Check sheet for the drawn part. Datum: minimum x, y, z corner. Units: mm. A direction names the side the tool comes from. Give positions to 0.01 mm unless a question says otherwise; leave off trailing zeros. Write each loop counter-clockwise with the first axis right and the second up, starting at its lowest first coordinate (ties: lowest second). Pieces come first, ordered by that corner, then holes. Notation, with made-up numbers: (35, 15.25) -> (90, 15.25) arc R29 ccw to (90, 54.25) -> close; hole circle Ø7 at (-39, -10). An arc over 180 degrees is marked (long way). Write item = value, one per line. Start each with the question number.
1. Mould release check, pull along Y, two halves, no side actions. Record for the marked faces 1, 2 and 3: pulls with the +Y half, pulls with the -Y half, needs draft (parallel to the pull), parting line crosses it, or undercut.
2. Set-up check for the marked faces 4, 5 and 6: record each of +Z, -Z, +X, -X, +Y, -Y from which the full face is reachable in a straight line by a thin tool's end or side.
3. Depth check by flat-ended pin: P1, Ø1, axis at x = 42.5, z = 46, coming from the +Y side; P2, Ø4, axis at x = 22.5, z = 49.5, coming from the +Y side; P3, Ø7.5, axis at x = 54.5, z = 38.5, coming from the +Y side; P4, Ø19, axis at y = 56.5, z = 32, coming from the +X side. Enter the tip coordinate at first touch or a pass-through.
4. Cross-section at D-D, the plane x = 50.8. Record the cut outline in (y, z) (3 decimals).
5. Thickness scan on line 1 along X through (y, z) = (3, 31.75) (3 decimals); line 2 along Y through (x, z) = (37.5, 35) (3 decimals); line 3 along X through (y, z) = (1, 31) (3 decimals). Record the ranges inside material, lowest first.
6. Cross-section at C-C, the plane y = 54. Record the cut outline in (x, z) (1 decimal), plus the area to 3 significant figures.
7. Cross-section at B-B, the plane x = 40. Record the cut outline in (y, z) (3 decimals).
8. Cross-section at A-A, the plane z = 38.5. Record the cut outline in (x, y) (3 decimals), plus the area to 3 significant figures.
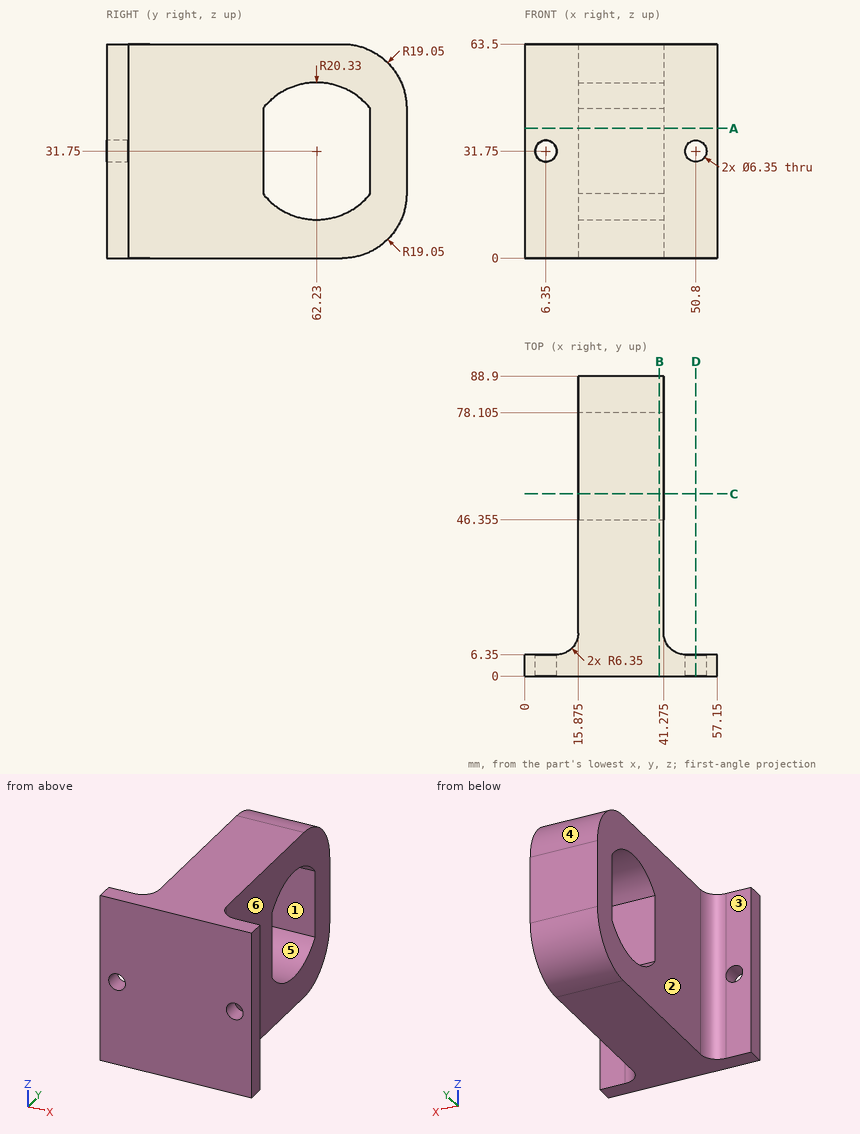
Answers:
q1.face_1 = undercut
q1.face_2 = needs draft
q1.face_3 = pulls with the +Y half
q2.face_4 = +Z, +X, -X, +Y
q2.face_5 = +X, -X
q2.face_6 = +Z, -Z, +X, +Y
q3.P1 = 9.75
q3.P2 = 88.65
q3.P3 = 6.35
q3.P4 = through
q4.outline = (0, 0) -> (6.35, 0) -> (6.35, 28.575) -> (0, 28.575) -> close; (0, 34.925) -> (6.35, 34.925) -> (6.35, 63.5) -> (0, 63.5) -> close
q5.line_1 = 0 to 3.175, 9.525 to 47.625, 53.975 to 57.15
q5.line_2 = 0 to 46.355, 78.105 to 88.9
q5.line_3 = 0 to 3.265, 9.435 to 47.715, 53.885 to 57.15
q6.outline = (15.9, 0) -> (41.3, 0) -> (41.3, 13.2) -> (15.9, 13.2) -> close; (15.9, 50.3) -> (41.3, 50.3) -> (41.3, 63.5) -> (15.9, 63.5) -> close
q6.area = 669 mm^2
q7.outline = (0, 0) -> (69.85, 0) arc R19.05 ccw to (88.9, 19.05) -> (88.9, 44.45) arc R19.05 ccw to (69.85, 63.5) -> (0, 63.5) -> close; hole (46.355, 19.05) arc R20.33 ccw to (78.105, 19.05) -> (78.105, 44.45) arc R20.33 ccw to (46.355, 44.45) -> close
q8.outline = (0, 0) -> (57.15, 0) -> (57.15, 6.35) -> (47.625, 6.35) arc R6.35 cw to (41.275, 12.7) -> (41.275, 46.355) -> (15.875, 46.355) -> (15.875, 12.7) arc R6.35 cw to (9.525, 6.35) -> (0, 6.35) -> close; (15.875, 78.105) -> (41.275, 78.105) -> (41.275, 88.9) -> (15.875, 88.9) -> close
q8.area = 1,670 mm^2
